Work out the finished part from the listing and answer in its coordinate system (mm). Round coordinates to 2 decimals unless told otherwise and drop trailing zeros. Write each loop counter-clockwise with the first axis right and the second up, starting at its lowest first coordinate (ties: lowest second). Pieces come first, ordered by that corner, then holes. Notation, with made-up numbers: (61.25, 12) -> (86.25, 12) arc R25 cw to (86.25, 38) -> close; hole circle Ø1 at (35.5, -16). An arc over 180 degrees is marked (long way). Answer as a JSON object with one key per item and string values. Group by question number.
from build123d import *

# Parameters (mm, degrees)
F1_DEPTH = 2
F2_R     = 2.5
F2_R_2   = 2.05
F3_DEPTH = 25
F4_R     = 5
F6_DEPTH = 25


with BuildPart() as f1:
    # F0 (on Front) → F1 (new body)
    with BuildSketch(Plane.XZ):
        Polygon((0, 180), (-760, 180), (-760, 130), (-460, 130), (-80, 0), (0, 0), align=None)
    extrude(amount=F1_DEPTH)

    # F2 (on face) → F3 (cut)
    with BuildSketch(Plane.XZ.offset(2)):
        with Locations((-15, 25)):
            Circle(F2_R)
        with Locations((-45, 25)):
            Circle(F2_R)
        with Locations((-265, 165)):
            Circle(F2_R)
        with Locations((-505, 165)):
            Circle(F2_R)
        with Locations((-745, 165)):
            Circle(F2_R)
        with Locations((-347.617717, 123.260407)):
            Circle(F2_R)
        with Locations((-319.232797, 113.549776)):
            Circle(F2_R)
        with Locations((-158.38492, 58.522871)):
            Circle(F2_R)
        with Locations((-130, 48.81224)):
            Circle(F2_R)
        with Locations((-625, 140)):
            Circle(F2_R)
        with Locations((-595, 140)):
            Circle(F2_R)
        with Locations((-15, 125)):
            Circle(F2_R)
        with Locations((-45, 125)):
            Circle(F2_R)
        with Locations((-740, 140)):
            Circle(F2_R_2)
        with Locations((-480, 140)):
            Circle(F2_R_2)
        with Locations((-437.839844, 132.987886)):
            Circle(F2_R_2)
        with Locations((-248.607047, 68.25035)):
            Circle(F2_R_2)
        with Locations((-95.686403, 15.935393)):
            Circle(F2_R_2)
        with Locations((-10, 90)):
            Circle(F2_R_2)
        with BuildLine():
            Line((-720.5, 161.5), (-709.5, 161.5))
            ThreePointArc((-709.5, 161.5), (-706, 165), (-709.5, 168.5))
            Line((-709.5, 168.5), (-720.5, 168.5))
            ThreePointArc((-720.5, 168.5), (-724, 165), (-720.5, 161.5))
        make_face()
        with BuildLine():
            Line((-41.5, 144.5), (-41.5, 155.5))
            ThreePointArc((-41.5, 155.5), (-45, 159), (-48.5, 155.5))
            Line((-48.5, 155.5), (-48.5, 144.5))
            ThreePointArc((-48.5, 144.5), (-45, 141), (-41.5, 144.5))
        make_face()
        with BuildLine():
            Line((-385.5, 161.5), (-374.5, 161.5))
            ThreePointArc((-374.5, 161.5), (-371, 165), (-374.5, 168.5))
            Line((-374.5, 168.5), (-385.5, 168.5))
            ThreePointArc((-385.5, 168.5), (-389, 165), (-385.5, 161.5))
        make_face()
        with BuildLine():
            Line((-11.5, 144.5), (-11.5, 155.5))
            ThreePointArc((-11.5, 155.5), (-15, 159), (-18.5, 155.5))
            Line((-18.5, 155.5), (-18.5, 144.5))
            ThreePointArc((-18.5, 144.5), (-15, 141), (-11.5, 144.5))
        make_face()
        with BuildLine():
            Line((-41.5, 49.5), (-41.5, 60.5))
            ThreePointArc((-41.5, 60.5), (-45, 64), (-48.5, 60.5))
            Line((-48.5, 60.5), (-48.5, 49.5))
            ThreePointArc((-48.5, 49.5), (-45, 46), (-41.5, 49.5))
        make_face()
        with BuildLine():
            Line((-11.5, 49.5), (-11.5, 60.5))
            ThreePointArc((-11.5, 60.5), (-15, 64), (-18.5, 60.5))
            Line((-18.5, 60.5), (-18.5, 49.5))
            ThreePointArc((-18.5, 49.5), (-15, 46), (-11.5, 49.5))
        make_face()
    extrude(amount=-F3_DEPTH, mode=Mode.SUBTRACT)

    # F4
    f4_edges = [f1.edges().sort_by_distance(p)[0] for p in [
        (-760, -1, 180),
        (-760, -1, 130),
        (-460, -1, 130),
        (-80, -1, 0),
        (0, -1, 0),
        (0, -1, 180),
    ]]
    fillet(f4_edges, radius=F4_R)

    # F5 (on face) → F6 (cut)
    with BuildSketch(Plane.XZ.offset(2)):
        Polygon((-60, 150), (-315, 150), (-315, 120), (-110.384615, 50), (-60, 50), align=None)
    extrude(amount=-F6_DEPTH, mode=Mode.SUBTRACT)


solid = f1.part
1) A cutting plane is placed at B-B on x = -407.5. Determine the outline of the cut face in (y, z), plus the area to 3 significant figures.
2) A cutting plane is placed at A-A on x = -276. Determine the outline of the cut face in (y, z), plus the area to 3 significant figures.
3) Each of these flat-tipped pins is pushed along its axis until it touches: P1, Ø0.6, axis at x = -639, y = -1, coming from the -Z side; P2, Ø1, axis at x = -226, y = -1, coming from the -Z side. Where does it stop, or does it pass through?
4) For a pull along Z with two mould halves and no side action, classify faces 1 (the face through (-214.12, -1.01, 85.49)), 2 (the face through (-272.649, -0.986, 65.906)), 3 (the face through (-301, -2, 111)) as released by +Z, released by -Z, zero draft, split by the parting line, or undercut.
5) Straight lines are drawn through the part: L1, parallel to X at y = -1.65, z = 150.5; L2, parallel to Z at x = -45, y = -1.2; L3, parallel to X at y = -1.55, z = 140. For each, find the intervals that lie inside material, in ascending order.
6) A cutting plane is placed at C-C on y = -0.5. State how many separate pieces and enclosed holes the cut face has, plus the area to 3 significant figures.
7) A cutting plane is placed at D-D on x = -670. Determine the outline of the cut face in (y, z), plus the area to 3 significant figures.
Established:
{
 "1": {"outline": "(-2, 112.04) -> (0, 112.04) -> (0, 180) -> (-2, 180) -> close", "area": "136 mm²"},
 "2": {"outline": "(-2, 67.05) -> (0, 67.05) -> (0, 106.66) -> (-2, 106.66) -> close; (-2, 150) -> (0, 150) -> (0, 180) -> (-2, 180) -> close", "area": "139 mm²"},
 "3": {"P1": "stops at z = 130", "P2": "stops at z = 49.78"},
 "4": {"face 1": "undercut", "face 2": "released by -Z", "face 3": "zero draft"},
 "5": {"L1": "x = -760 to -48.5, -41.5 to -18.5, -11.5 to 0", "L2": "z = 0 to 22.5, 27.5 to 46, 64 to 122.5, 127.5 to 141, 159 to 180", "L3": "x = -760 to -742.05, -737.95 to -627.5, -622.5 to -597.5, -592.5 to -482.05, -477.95 to -315, -60 to 0"},
 "6": {"separate pieces": "1", "enclosed holes": "26", "area": "53,700 mm²"},
 "7": {"outline": "(-2, 130) -> (0, 130) -> (0, 180) -> (-2, 180) -> close", "area": "100 mm²"}
}
